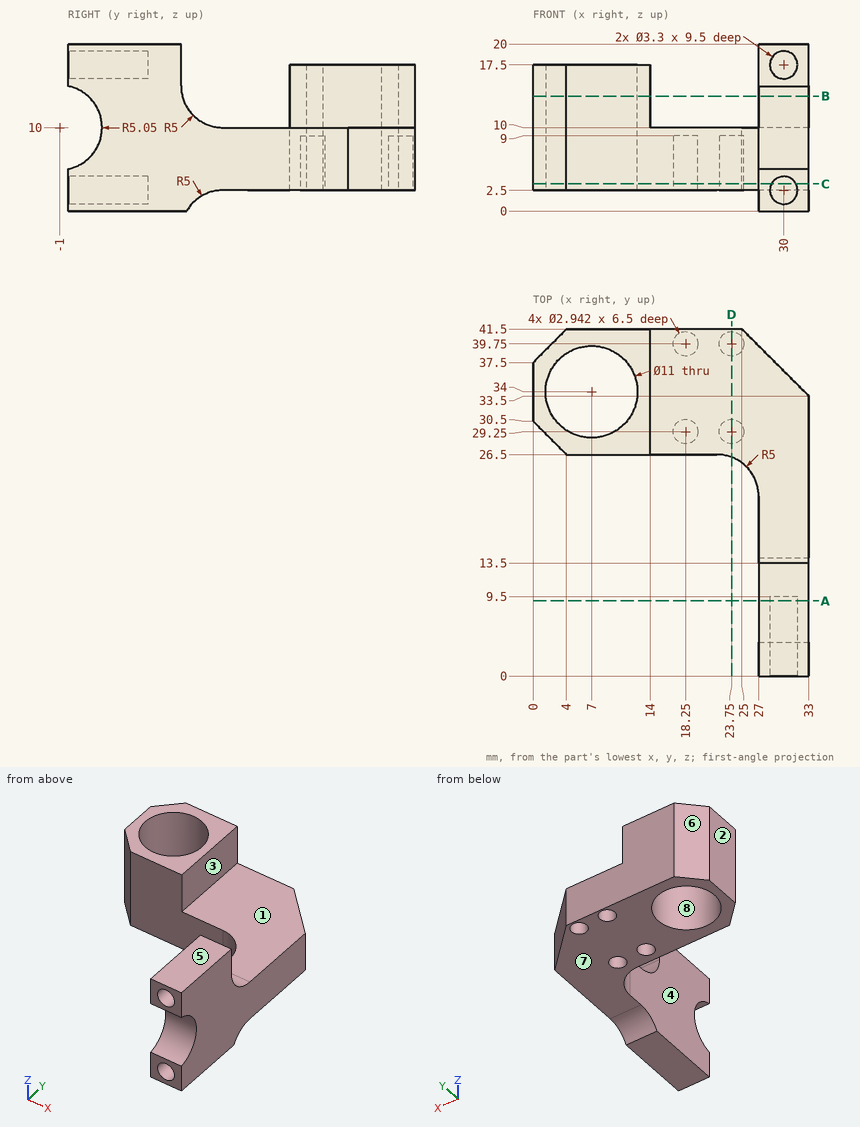
Check sheet for the drawn part. Datum: minimum x, y, z corner. Units: mm. A direction names the side the tool comes from. Coordinates: 2 decimals unless noted, no trailing zeros. Loops run counter-clockwise (first coordinate to the right, second up) from the corner with the lowest first, then second, coordinate; pieces in that order, holes last. Notation, with made-up numbers: (44.5, 8) -> (59.5, 8) arc R20 ccw to (59.5, 29) -> close; hole circle Ø1 at (-12.75, -16). An arc over 180 degrees is marked (long way). Answer in a Markdown table with one row per item.
1) Scan lines: line 1 along Y through (x, z) = (18.25, 5.75); line 2 along Z through (x, y) = (30, 5.75); line 3 along Y through (x, z) = (7, 12.75). Record each from-to range of solid material in increasing order. Write a range as from..to.
The answers:
| item | result |
|---|---|
| line 1 | y = 26.5..27.78, 30.72..38.28, 41.22..41.5 |
| line 2 | z = 0..0.85, 4.15..15.85, 19.15..20 |
| line 3 | y = 26.5..28.5, 39.5..41.5 |
2) Section check B-B (z = 13.75). Record the cut outline in (x, y), and give its area (3 significant figures).
The answers:
| item | result |
|---|---|
| outline | (0, 30.5) -> (4, 26.5) -> (14, 26.5) -> (14, 41.5) -> (4, 41.5) -> (0, 37.5) -> close; (27, 2.38) -> (33, 2.38) -> (33, 13.66) -> (27, 13.66) -> close; hole circle Ø11 at (7, 34) |
| area | 167 mm2 |
3) Section check A-A (y = 9). Record the cut outline in (x, z).
The answers:
| item | result |
|---|---|
| outline | (27, 0) -> (33, 0) -> (33, 20) -> (27, 20) -> close; hole circle Ø3.3 at (30, 2.5); hole circle Ø3.3 at (30, 17.5) |
4) Draft check along X on the marked faces 6, 7 and 8. Enter one of: released by +X, released by -X, zero draft, split by the parting line, or undercut.
The answers:
| item | result |
|---|---|
| face 6 | released by -X |
| face 7 | zero draft |
| face 8 | undercut |
5) Access from +Z, -Z, +X, -X, +Y, -Y to the whole of each face (thin tool, end or side, straight path). Record for the marked faces 1, 2, 3, 4 and 5.
The answers:
| item | result |
|---|---|
| face 1 | +Z, +X, +Y |
| face 2 | +Z, -Z, -X, +Y, -Y |
| face 3 | +Z, +X, +Y, -Y |
| face 4 | +Z, -Z, -X, -Y |
| face 5 | +Z, +X, -X, +Y, -Y |
6) Depth check by flat-ended pin: P1, Ø5, axis at x = 14.5, z = 10, coming from the -Y side; P2, Ø8, axis at y = 13.5, z = 8, coming from the -X side; P3, Ø3, axis at x = 23.5, y = 40, coming from the -Z side. Enter the tip coordinate at first touch or a pass-through.
The answers:
| item | result |
|---|---|
| P1 | stops at y = 26.5 |
| P2 | stops at x = 27 |
| P3 | stops at z = 2.5 |
7) Section check C-C (z = 3.25). Record the cut outline in (x, y).
The answers:
| item | result |
|---|---|
| outline | (0, 30.5) -> (4, 26.5) -> (22, 26.5) arc R5 cw to (27, 21.5) -> (27, 0) -> (28.53, 0) -> (28.53, 9.5) -> (31.47, 9.5) -> (31.47, 0) -> (33, 0) -> (33, 33.5) -> (25, 41.5) -> (4, 41.5) -> (0, 37.5) -> close; hole circle Ø11 at (7, 34); hole circle Ø2.94 at (18.25, 29.25); hole circle Ø2.94 at (18.25, 39.75); hole circle Ø2.94 at (23.75, 29.25); hole circle Ø2.94 at (23.75, 39.75) |
8) Section check D-D (x = 23.75). Record the cut outline in (y, z).
The answers:
| item | result |
|---|---|
| outline | (26.18, 2.5) -> (27.78, 2.5) -> (27.78, 9) -> (30.72, 9) -> (30.72, 2.5) -> (38.28, 2.5) -> (38.28, 9) -> (41.22, 9) -> (41.22, 2.5) -> (41.5, 2.5) -> (41.5, 10) -> (26.18, 10) -> close |
